Check sheet for the drawn part. Datum: minimum x, y, z corner. Units: mm. A direction names the side the tool comes from. Give positions to 0.01 mm unless a question says otherwise; leave off trailing zeros. Order: outer loops, then holes, each group sorted by start corner. A loop starts at its lowest first (then second) coordinate and runs counter-clockwise, first axis right, second up.
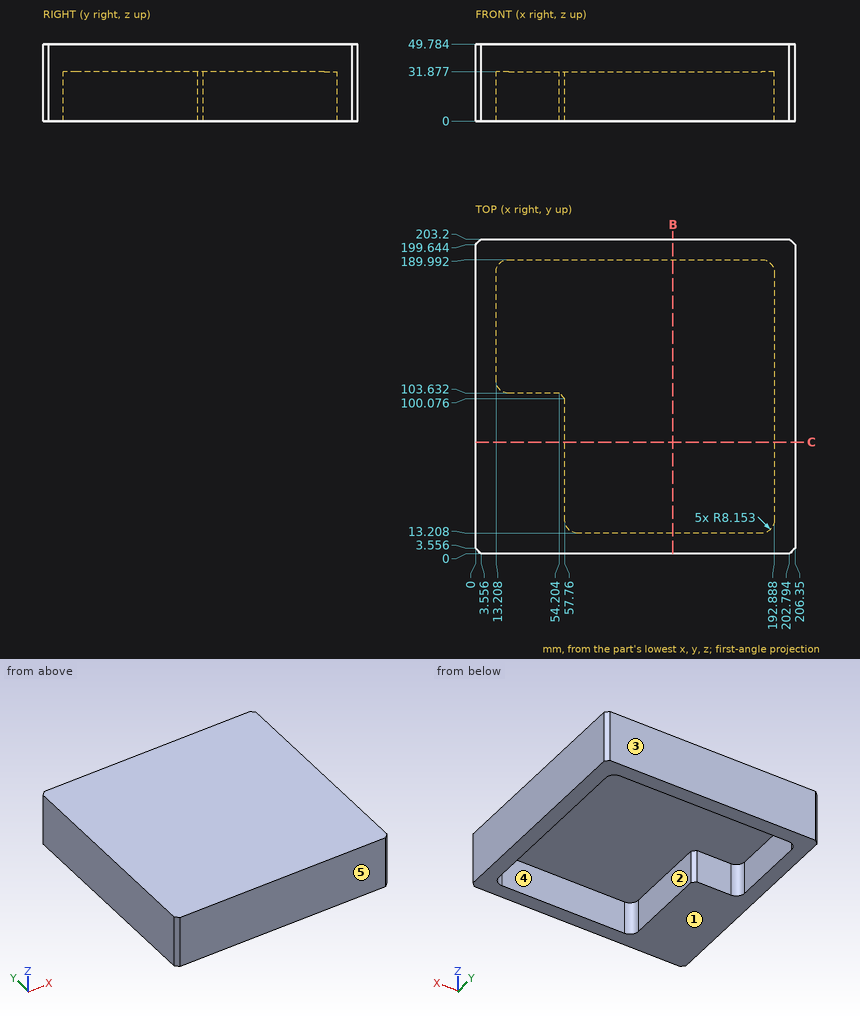
Q1. Material ranges on line 1 (X direction, y = 33, z = 20.5); line 2 (X direction, y = 139, z = 27); line 3 (Y direction, x = 162, z = 30), recorded low to high.
Q2. Sectioned sample at C-C, the plane y = 72. Record the cut outline in (x, z).
Q3. Sectioned sample at B-B, the plane x = 127.5. Record the cut outline in (y, z).
Q4. Tool access check on the marked faces 1 and 2. Record the directions out of +Z, -Z, +X, -X, +Y, -Y that give a thin tool (end or side, any length) a straight path to the whole face; none if there is none.
Q5. Draft check along Y on the marked faces 3, 4 and 5. Enter one of: pulls with the +Y half, pulls with the -Y half, needs draft (parallel to the pull), parting line crosses it, or undercut.
Filled in:
1. line 1: x = 0 to 57.76, 192.89 to 206.35
1. line 2: x = 0 to 13.21, 192.89 to 206.35
1. line 3: y = 0 to 13.21, 189.99 to 203.2
2. outline: (0, 0) - (57.76, 0) - (57.76, 31.88) - (192.89, 31.88) - (192.89, 0) - (206.35, 0) - (206.35, 49.78) - (0, 49.78) - close
3. outline: (0, 0) - (13.21, 0) - (13.21, 31.88) - (189.99, 31.88) - (189.99, 0) - (203.2, 0) - (203.2, 49.78) - (0, 49.78) - close
4. face 1: -Z, +X, -X, +Y, -Y
4. face 2: -Z
5. face 3: pulls with the +Y half
5. face 4: undercut
5. face 5: pulls with the -Y half
